from build123d import *

# Parameters (mm, degrees)
SKETCH014_R  = 2.2
PAD010_DEPTH = 1.8
SKETCH016_W  = 25
SKETCH016_H  = 15
SKETCH025_W  = 18
SKETCH025_H  = 15
SKETCH017_W  = 6.5
SKETCH017_H  = 15
SKETCH018_R  = 1.75
PAD011_DEPTH = 3.25
SKETCH015_W  = 28
SKETCH015_H  = 6
PAD012_DEPTH = 2.5


with BuildPart() as part:
    # Sketch014 → Pad010 (new body)
    with BuildSketch(Plane.XY):
        with BuildLine():
            Line((-25.5, 7.5), (25.5, 7.5))
            ThreePointArc((27.5, 5.5), (26.914214, 6.914214), (25.5, 7.5))
            Line((27.5, 5.5), (27.5, -5.5))
            ThreePointArc((25.5, -7.5), (26.914214, -6.914214), (27.5, -5.5))
            Line((25.5, -7.5), (-25.5, -7.5))
            ThreePointArc((-27.5, -5.5), (-26.914214, -6.914214), (-25.5, -7.5))
            Line((-27.5, -5.5), (-27.5, 5.5))
            ThreePointArc((-25.5, 7.5), (-26.914214, 6.914214), (-27.5, 5.5))
        make_face()
        with Locations((-20, 0)):
            Circle(SKETCH014_R, mode=Mode.SUBTRACT)
        with Locations((20, 0)):
            Circle(SKETCH014_R, mode=Mode.SUBTRACT)
    extrude(amount=-PAD010_DEPTH)

    # Sketch016 → AdditiveLoft section 0
    with BuildSketch(Plane.XY):
        Rectangle(SKETCH016_W, SKETCH016_H)
    # Sketch025 → AdditiveLoft section 1
    with BuildSketch(Plane.XY.offset(5)):
        Rectangle(SKETCH025_W, SKETCH025_H)
    # Sketch017 → AdditiveLoft section 2
    with BuildSketch(Plane.XY.offset(25)):
        Rectangle(SKETCH017_W, SKETCH017_H)
    loft()

    # Sketch018 → Pad011 (join, symmetric)
    with BuildSketch(Plane(origin=(0, 0, 25), x_dir=(0, 1, 0), z_dir=(1, 0, 0))):
        with BuildLine():
            Line((7.5, 0), (-7.5, 0))
            Line((-7.5, 0), (-7.5, 9))
            ThreePointArc((7.5, 9), (0, 16.5), (-7.5, 9))
            Line((7.5, 9), (7.5, 0))
        make_face()
        with Locations((0, 9)):
            Circle(SKETCH018_R, mode=Mode.SUBTRACT)
    extrude(amount=PAD011_DEPTH, both=True)

    # Sketch015 → Pad012 (join)
    with BuildSketch(Plane(origin=(0, 0, -1.8), x_dir=(1, 0, 0), z_dir=(0, 0, -1))):
        Rectangle(SKETCH015_W, SKETCH015_H)
    extrude(amount=PAD012_DEPTH)


solid = part.part
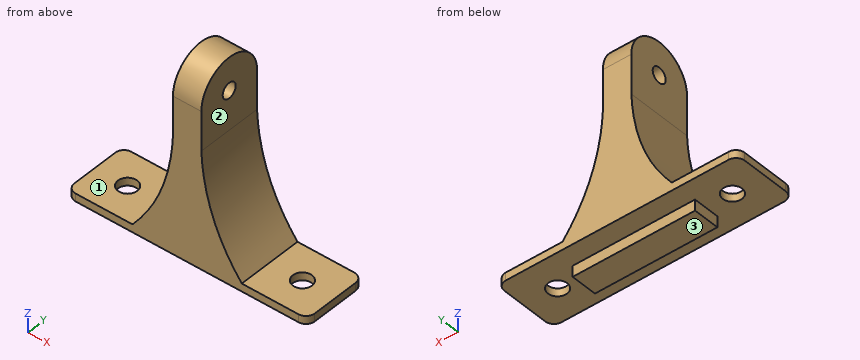
The model under review builds one solid part; all positions refer to its coordinate system, in mm. Face numbers are marked on the shaded views. A direction names the side the tool comes from. Coordinates: 2 decimals unless noted, no trailing zeros. Loops run counter-clockwise (first coordinate to the right, second up) from the corner with the lowest first, then second, coordinate; pieces in that order, holes last. Notation, with made-up numbers: M 10.25,3.5 L 21.25,3.5 A16 ccw 21.25,11.5 Z; hole C -16,39 d1. An arc over 180 degrees is marked long. Put each result on its own line as item: value. Start each with the question number.
Q1. Clearance check with flat-ended pins moving along their axes: pin 1 (4 mm diameter, centred on y = 2.5, z = 33.5, fed in from -X); pin 2 (1.5 mm diameter, centred on y = 0.5, z = 29, fed in from +X); pin 3 (2 mm diameter, centred on x = 6, z = -3.5, fed in from +Y). State where each tip first meets the part, or that it passes through.
Q2. Add section A-A (x = 20). Write out the cut boundary in (y, z), and give its area (3 significant figures).
Q3. Add section C-C (x = -17). Write out the cut boundary in (y, z), and give its area (3 significant figures).
Q4. Add section B-B (y = 0). Count the separate pieces of the cut face and the enclosed holes in it, and give its area (3 significant figures).
Q5. Wall thickness on line 1 (Y direction, x = -20, z = -1); line 2 (X direction, y = 3.25, z = 38.5); line 3 (Z direction, x = 18, y = 4.75): over which ranges is each line inside the solid? List them lowest first.
Q6. For the marked faces 1, 2 and 3, list the 3-axis set-ups (+Z, -Z, +X, -X, +Y, -Y) from which the entire face can be reached by the end or side of a thin tool; tool diameter is ignored.
Q7. Add section D-D (z = 36.5). Write out the cut boundary in (x, y).
Answers:
1. pin 1: stops at x = -3.25
1. pin 2: stops at x = 3.25
1. pin 3: stops at y = 3
2. outline: M -7.5,-1.8 L -2.2,-1.8 L -2.2,0 L -7.5,0 Z; M 2.2,-1.8 L 7.5,-1.8 L 7.5,0 L 2.2,0 Z
2. area: 19.1 mm^2
3. outline: M -7.5,-1.8 L 7.5,-1.8 L 7.5,0 L -7.5,0 Z
3. area: 27.0 mm^2
4. separate pieces: 4
4. enclosed holes: 0
4. area: 553 mm^2
5. line 1: y = -7.5 to -2.2, 2.2 to 7.5
5. line 2: x = -3.25 to 3.25
5. line 3: z = -1.8 to 0
6. face 1: +Z, -X, +Y, -Y
6. face 2: +Z, +X, +Y, -Y
6. face 3: -Z, +X, -X, +Y, -Y
7. outline: M -3.25,-7.07 L 3.25,-7.07 L 3.25,7.07 L -3.25,7.07 Z
